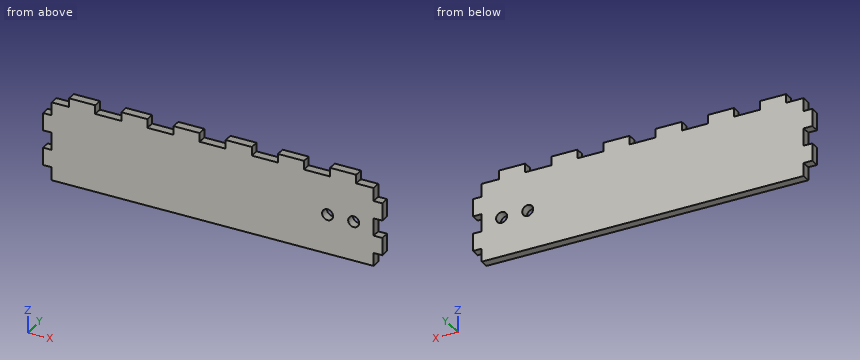
from build123d import *

# Parameters (mm, degrees)
ESQUISSE1_W                     = 234.95
ESQUISSE1_H                     = 57.15
BOSS_EXTRU_1_DEPTH              = 6.35
ESQUISSE3_W                     = 19.05
ESQUISSE3_H                     = 6.35
BOSS_EXTRU_2_DEPTH              = 6.35
R_P_TITION_LIN_AIRE2_COUNT      = 6
R_P_TITION_LIN_AIRE2_PITCH      = 38.1
ESQUISSE5_W                     = 6.35
ESQUISSE5_H                     = 12.7
BOSS_EXTRU_4_DEPTH              = 6.35
R_P_TITION_LIN_AIRE4_COUNT      = 2
R_P_TITION_LIN_AIRE4_PITCH      = 25.4
R_P_TITION_LIN_AIRE4_COUNT_DIR2 = 2
R_P_TITION_LIN_AIRE4_PITCH_DIR2 = 241.3
ESQUISSE2_R                     = 4
ENL_V_MAT_EXTRU_1_DEPTH         = 6.35


with BuildPart() as part:
    # Esquisse1 → Boss.-Extru.1 (new body)
    with BuildSketch(Plane(origin=(0, 0, 0), x_dir=(1, 0, 0), z_dir=(0, 1, 0))):
        Rectangle(ESQUISSE1_W, ESQUISSE1_H)
    extrude(amount=BOSS_EXTRU_1_DEPTH)

    # Esquisse3 → Boss.-Extru.2 (add)
    with BuildSketch(Plane(origin=(0, 6.35, 0), x_dir=(1, 0, 0), z_dir=(0, 1, 0))):
        with Locations((-95.25, -31.75)):
            Rectangle(ESQUISSE3_W, ESQUISSE3_H)
    boss_extru_2 = extrude(amount=-BOSS_EXTRU_2_DEPTH)

    # Répétition linéaire2: Boss.-Extru.2 ×6
    with Locations(*[(i * R_P_TITION_LIN_AIRE2_PITCH, 0, 0) for i in range(1, R_P_TITION_LIN_AIRE2_COUNT)]):
        add(boss_extru_2)

    # Esquisse5 → Boss.-Extru.4 (add)
    with BuildSketch(Plane(origin=(0, 6.35, 0), x_dir=(1, 0, 0), z_dir=(0, 1, 0))):
        with Locations((-120.65, -12.7)):
            Rectangle(ESQUISSE5_W, ESQUISSE5_H)
    boss_extru_4 = extrude(amount=-BOSS_EXTRU_4_DEPTH)

    # Répétition linéaire4: Boss.-Extru.4 2 × 2
    with Locations(*[(j * R_P_TITION_LIN_AIRE4_PITCH_DIR2, 0, -i * R_P_TITION_LIN_AIRE4_PITCH) for i in range(R_P_TITION_LIN_AIRE4_COUNT) for j in range(R_P_TITION_LIN_AIRE4_COUNT_DIR2) if (i, j) != (0, 0)]):
        add(boss_extru_4)

    # Esquisse2 → Enlèv. mat.-Extru.1 (cut)
    with BuildSketch(Plane(origin=(0, 6.35, 0), x_dir=(1, 0, 0), z_dir=(0, 1, 0))):
        with Locations(Location((83.895833333, 0, 0), (0, 0, 270))):
            Circle(ESQUISSE2_R)
        with Locations(Location((102.945833333, 0, 0), (0, 0, 270))):
            Circle(ESQUISSE2_R)
    extrude(amount=-ENL_V_MAT_EXTRU_1_DEPTH, mode=Mode.SUBTRACT)


solid = part.part
The listing builds one solid part. Answer for the finished solid, in the listing's coordinates (mm). Give positions to 0.01 mm unless a question says otherwise; leave off trailing zeros. Write each loop counter-clockwise with the first axis right and the second up, starting at its lowest first coordinate (ties: lowest second). Pieces come first, ordered by that corner, then holes.
Item 1: Flat-ended cylindrical pins translate along their axes: P1, Ø1.5, axis at y = 2.5, z = 1.5, coming from the -X side (3 decimals); P2, Ø7, axis at x = 83.9, z = 0, coming from the +Y side; P3, Ø1.9, axis at y = 3, z = 30.5, coming from the -X side (3 decimals); P4, Ø1.9, axis at x = -121.5, y = 2.5, coming from the -Z side. Find the tip coordinate at first contact, or state that the pin passes through.
Item 2: Section C-C, the plane x = 1 is taken. Write down the section's boundary in (y, z) (3 decimals), plus the area to 3 significant figures.
Item 3: Find the intervals of material crossed by line 1 along X through (y, z) = (5.25, 0) (3 decimals); line 2 along X through (y, z) = (5, 3.5) (3 decimals); line 3 along X through (y, z) = (3.5, -6) (3 decimals), in increasing order.
Item 4: Section D-D, the plane y = 2.5 is taken. Count the separate pieces of the cut face and the enclosed holes in it, plus the area to 3 significant figures.
Item 5: Section A-A, the plane z = 0 is taken. Write down the section's boundary in (x, y) (3 decimals).
Item 6: Section B-B, the plane z = 31.5 is taken. Write down the section's boundary in (x, y) (3 decimals).
Completed:
1. P1: stops at x = -117.475
1. P2: passes through
1. P3: stops at x = -104.775
1. P4: stops at z = -19.05
2. outline: (0, -28.575) - (6.35, -28.575) - (6.35, 28.575) - (0, 28.575) - close
2. area: 363 mm2
3. line 1: x = -117.475 to 79.896, 87.896 to 98.946, 106.946 to 117.475
3. line 2: x = -117.475 to 81.959, 85.832 to 101.009, 104.882 to 117.475
3. line 3: x = -117.475 to 117.475
4. separate pieces: 1
4. enclosed holes: 2
4. area: 14,400 mm2
5. outline: (-117.475, 0) - (79.896, 0) - (79.896, 6.35) - (-117.475, 6.35) - close; (87.896, 0) - (98.946, 0) - (98.946, 6.35) - (87.896, 6.35) - close; (106.946, 0) - (117.475, 0) - (117.475, 6.35) - (106.946, 6.35) - close
6. outline: (-104.775, 0) - (-85.725, 0) - (-85.725, 6.35) - (-104.775, 6.35) - close; (-66.675, 0) - (-47.625, 0) - (-47.625, 6.35) - (-66.675, 6.35) - close; (-28.575, 0) - (-9.525, 0) - (-9.525, 6.35) - (-28.575, 6.35) - close; (9.525, 0) - (28.575, 0) - (28.575, 6.35) - (9.525, 6.35) - close; (47.625, 0) - (66.675, 0) - (66.675, 6.35) - (47.625, 6.35) - close; (85.725, 0) - (104.775, 0) - (104.775, 6.35) - (85.725, 6.35) - close
